For this review, take the finished solid that the model builds, in its own axes (mm). Face numbers are marked on the shaded views. Coordinates: 2 decimals unless noted, no trailing zeros. Order: outer loops, then holes, each group sorted by start corner. A loop starts at its lowest first (then second) coordinate and runs counter-clockwise, first axis right, second up.
from build123d import *

# Parameters (mm, degrees)
SKETCH1_W           = 127.75
SKETCH1_H           = 85.6
BOSS_EXTRUDE1_DEPTH = 14.35
FILLET1_R           = 3
CUT_FLANGE_DEPTH    = 8.25
SKETCH5_W           = 80.1
SKETCH5_H           = 0.75
CUT_PAPERSLOT_DEPTH = 123.75
SHELL1_DEPTH        = 11.1
SHELL1_2_DEPTH      = 5.1
SKETCH4_W           = 8.5
SKETCH4_H           = 8.5
CUT_EXTRUDE3_DEPTH  = 20


# Read off the part's stored shape, not the designer's step: Shell1
with BuildPart() as part:
    # Sketch1 → Boss-Extrude1 (new body)
    with BuildSketch(Plane(origin=(0, 0, 0), x_dir=(1, 0, 0), z_dir=(0, 1, 0))):
        Rectangle(SKETCH1_W, SKETCH1_H)
    extrude(amount=BOSS_EXTRUDE1_DEPTH)

    # Fillet1
    fillet1_edges = [part.edges().sort_by_distance(p)[0] for p in [
        (-63.875, 7.175, -42.8),
        (63.875, 7.175, -42.8),
        (63.875, 7.175, 42.8),
        (-63.875, 7.175, 42.8),
    ]]
    fillet(fillet1_edges, radius=FILLET1_R)

    # Sketch3 → Cut-Flange (cut)
    with BuildSketch(Plane(origin=(0, 14.35, 0), x_dir=(1, 0, 0), z_dir=(0, 1, 0))):
        with BuildLine():
            Line((-63.875, 39.8), (-63.875, -39.8))
            ThreePointArc((-63.875, -39.8), (-62.996320344, -41.921320344), (-60.875, -42.8))
            Line((-60.875, -42.8), (60.875, -42.8))
            ThreePointArc((60.875, -42.8), (62.996320344, -41.921320344), (63.875, -39.8))
            Line((63.875, -39.8), (63.875, 39.8))
            ThreePointArc((63.875, 39.8), (62.996320344, 41.921320344), (60.875, 42.8))
            Line((60.875, 42.8), (-60.875, 42.8))
            ThreePointArc((-60.875, 42.8), (-62.996320344, 41.921320344), (-63.875, 39.8))
        make_face()
        with BuildLine():
            Line((-62.625, 36.600252532), (-62.625, -39.8))
            ThreePointArc((-62.625, -39.8), (-62.112436867, -41.037436867), (-60.875, -41.55))
            Line((-60.875, -41.55), (60.875, -41.55))
            ThreePointArc((60.875, -41.55), (62.112436867, -41.037436867), (62.625, -39.8))
            Line((62.625, -39.8), (62.625, 39.8))
            ThreePointArc((62.625, 39.8), (62.112436867, 41.037436867), (60.875, 41.55))
            Line((60.875, 41.55), (-57.675252532, 41.55))
            Line((-57.675252532, 41.55), (-62.625, 36.600252532))
        make_face(mode=Mode.SUBTRACT)
    extrude(amount=-CUT_FLANGE_DEPTH, mode=Mode.SUBTRACT)

    # Sketch5 → Cut-PaperSlot (cut)
    with BuildSketch(Plane.ZY.offset(62.625)):
        with Locations((0, 12.475)):
            Rectangle(SKETCH5_W, SKETCH5_H)
    extrude(amount=-CUT_PAPERSLOT_DEPTH, mode=Mode.SUBTRACT)

    # Shell1 outline → Shell1 (cut)
    with BuildSketch(Plane(origin=(0, 0, 0), x_dir=(1, 0, 0), z_dir=(0, 1, 0))):
        with BuildLine():
            Line((-61.625, 36.186038969), (-61.625, -39.8))
            ThreePointArc((-61.625, -39.8), (-61.405330086, -40.330330086), (-60.875, -40.55))
            Line((-60.875, -40.55), (60.875, -40.55))
            ThreePointArc((60.875, -40.55), (61.405330086, -40.330330086), (61.625, -39.8))
            Line((61.625, -39.8), (61.625, 39.8))
            ThreePointArc((61.625, 39.8), (61.405330086, 40.330330086), (60.875, 40.55))
            Line((60.875, 40.55), (-57.261038969, 40.55))
            Line((-57.261038969, 40.55), (-61.625, 36.186038969))
        make_face()
    extrude(amount=SHELL1_DEPTH, mode=Mode.SUBTRACT)

    # Shell1 2 outline → Shell1 2 (cut)
    with BuildSketch(Plane(origin=(0, 0, 0), x_dir=(1, 0, 0), z_dir=(0, 1, 0))):
        with BuildLine():
            Line((-62.875, 39.8), (-62.875, -39.8))
            ThreePointArc((-62.875, -39.8), (-62.289213562, -41.214213562), (-60.875, -41.8))
            Line((-60.875, -41.8), (60.875, -41.8))
            ThreePointArc((60.875, -41.8), (62.289213562, -41.214213562), (62.875, -39.8))
            Line((62.875, -39.8), (62.875, 39.8))
            ThreePointArc((62.875, 39.8), (62.289213562, 41.214213562), (60.875, 41.8))
            Line((60.875, 41.8), (-60.875, 41.8))
            ThreePointArc((-60.875, 41.8), (-62.289213562, 41.214213562), (-62.875, 39.8))
        make_face()
        with BuildLine():
            ThreePointArc((-60.875, -40.55), (-61.405330086, -40.330330086), (-61.625, -39.8))
            Line((-61.625, -39.8), (-61.625, 36.186038969))
            Line((-61.625, 36.186038969), (-57.261038969, 40.55))
            Line((-57.261038969, 40.55), (60.875, 40.55))
            ThreePointArc((60.875, 40.55), (61.405330086, 40.330330086), (61.625, 39.8))
            Line((61.625, 39.8), (61.625, -39.8))
            ThreePointArc((61.625, -39.8), (61.405330086, -40.330330086), (60.875, -40.55))
            Line((60.875, -40.55), (-60.875, -40.55))
        make_face(mode=Mode.SUBTRACT)
    extrude(amount=SHELL1_2_DEPTH, mode=Mode.SUBTRACT)

    # Sketch4 → Cut-Extrude3 (cut)
    with BuildSketch(Plane(origin=(0, 14.35, 0), x_dir=(1, 0, 0), z_dir=(0, 1, 0))):
        with Locations((-22.495, -13.44)):
            Rectangle(SKETCH4_W, SKETCH4_H)
    extrude(amount=-CUT_EXTRUDE3_DEPTH, mode=Mode.SUBTRACT)


solid = part.part
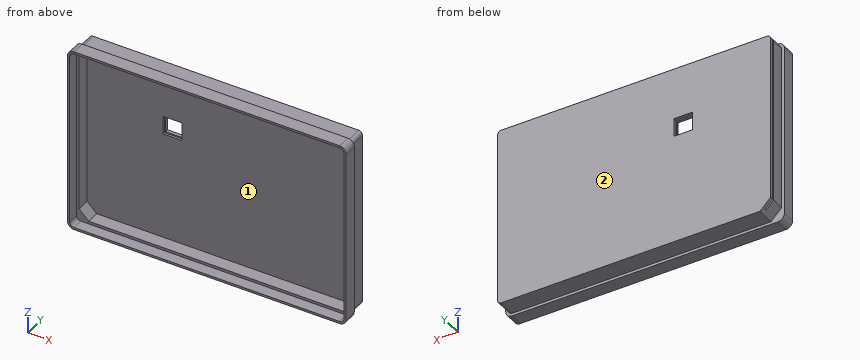
1. Clearance check with flat-ended pins moving along their axes: pin 1 Ø0.8 at (x, y) = (-23.5, 12) entering from +Z; pin 2 Ø1.1 at (y, z) = (11.5, 12.5) entering from +X (3 decimals); pin 3 Ø4 at (x, y) = (30, 11.5) entering from -Z. State where each tip first meets the part, or that it passes through.
Answer below:
pin 1: stops at z = 41.55
pin 2: stops at x = 62.625
pin 3: stops at z = -41.55
2. Take a section at B-B, the plane x = -31. Give the boundary of the cut face in (y, z), plus the area to 3 significant figures.
Answer below:
outline: (0, -42.8) - (6.1, -42.8) - (6.1, -41.55) - (14.35, -41.55) - (14.35, 41.55) - (6.1, 41.55) - (6.1, 42.8) - (0, 42.8) - (0, 41.8) - (5.1, 41.8) - (5.1, 40.55) - (11.1, 40.55) - (11.1, -40.55) - (5.1, -40.55) - (5.1, -41.8) - (0, -41.8) - close; hole (12.1, -40.05) - (12.85, -40.05) - (12.85, 40.05) - (12.1, 40.05) - close
area: 235 mm2
3. Take a section at D-D, the plane y = 2.5. Give the boundary of the cut face in (x, z) (3 decimals), plus the area to 3 significant figures.
Answer below:
outline: (-63.875, -39.8) arc R3 ccw to (-60.875, -42.8) - (60.875, -42.8) arc R3 ccw to (63.875, -39.8) - (63.875, 39.8) arc R3 ccw to (60.875, 42.8) - (-60.875, 42.8) arc R3 ccw to (-63.875, 39.8) - close; hole (-62.875, -39.8) arc R2 ccw to (-60.875, -41.8) - (60.875, -41.8) arc R2 ccw to (62.875, -39.8) - (62.875, 39.8) arc R2 ccw to (60.875, 41.8) - (-60.875, 41.8) arc R2 ccw to (-62.875, 39.8) - close
area: 418 mm2
4. Take a section at C-C, the plane z = -16. Give the boundary of the cut face in (x, y) (3 decimals).
Answer below:
outline: (-63.875, 0) - (-62.875, 0) - (-62.875, 5.1) - (-61.625, 5.1) - (-61.625, 11.1) - (61.625, 11.1) - (61.625, 5.1) - (62.875, 5.1) - (62.875, 0) - (63.875, 0) - (63.875, 6.1) - (62.625, 6.1) - (62.625, 14.35) - (-62.625, 14.35) - (-62.625, 12.85) - (61.125, 12.85) - (61.125, 12.1) - (-62.625, 12.1) - (-62.625, 6.1) - (-63.875, 6.1) - close
5. Take a section at A-A, the plane y = 9.5. Give the boundary of the cut face in (x, z) (3 decimals), plus the area to 3 significant figures.
Answer below:
outline: (-62.625, -36.6) - (-57.675, -41.55) - (60.875, -41.55) arc R1.75 ccw to (62.625, -39.8) - (62.625, 39.8) arc R1.75 ccw to (60.875, 41.55) - (-60.875, 41.55) arc R1.75 ccw to (-62.625, 39.8) - close; hole (-61.625, -36.186) - (-57.261, -40.55) - (60.875, -40.55) arc R0.75 ccw to (61.625, -39.8) - (61.625, 39.8) arc R0.75 ccw to (60.875, 40.55) - (-60.875, 40.55) arc R0.75 ccw to (-61.625, 39.8) - close
area: 408 mm2
6. To check wall thickness, follow L1, parallel to X at y = 4, z = -31.5 (3 decimals); L2, parallel to Z at x = -31.5, y = 9.75; L3, parallel to Y at x = 28, z = 3. State the ranges of each line that lie inside material, in increasing order.
Answer below:
L1: x = -63.875 to -62.875, 62.875 to 63.875
L2: z = -41.55 to -40.55, 40.55 to 41.55
L3: y = 11.1 to 12.1, 12.85 to 14.35
7. The part is to be moulded in two halves that separate along Z. For the marked faces 1 and 2, say which applies: +Z half, -Z half, draft (parallel to the pull), parting line (faces both ways), or undercut.
Answer below:
face 1: undercut
face 2: draft
